Build history of the part. All positions in model axes, mm. A direction names the side the tool comes from. Give positions to 0.01 mm unless a question says otherwise; leave off trailing zeros. Order: outer loops, then holes, each group sorted by start corner. A loop starts at its lowest first (then second) coordinate and runs counter-clockwise, first axis right, second up. Notation, with made-up numbers: (50.5, 27) -> (68.5, 27) arc R30 cw to (68.5, 51) -> close; hole circle Ø4 at (35.25, 87.25). An arc over 180 degrees is marked (long way). Use a Markdown table: item, result. Add a question column.
```python
from build123d import *

# Parameters (mm, degrees)
PAD_DEPTH    = 2.5
PAD001_DEPTH = 1.5
SKETCH002_R  = 2.5
PAD002_DEPTH = 25


with BuildPart() as part:
    # Sketch → Pad (new body, symmetric)
    with BuildSketch(Plane.XY):
        Polygon((-5, 0), (5, 0), (5, -1.284989), (2.784989, -3.5), (-2.784989, -3.5), (-5, -1.284989), align=None)
    extrude(amount=PAD_DEPTH, both=True)

    # Sketch001 → Pad001 (join)
    with BuildSketch(Plane.XZ):
        with BuildLine():
            ThreePointArc((-2.5, 0), (-1.767767, -1.767767), (0, -2.5))
            Line((0, -2.5), (2.5, -2.5))
            Line((2.5, 0), (2.5, -2.5))
            ThreePointArc((2.5, 0), (1.767767, 1.767767), (0, 2.5))
            Line((-2.5, 2.5), (0, 2.5))
            Line((-2.5, 0), (-2.5, 2.5))
        make_face()
    extrude(amount=-PAD001_DEPTH)

    # Sketch002 → Pad002 (join)
    with BuildSketch(Plane.XZ):
        Circle(SKETCH002_R)
    extrude(amount=-PAD002_DEPTH)


solid = part.part
```
(1) Band-saw the part on B-B on x = -1.5. Give the cut face in (y, z).
(2) Band-saw the part on A-A on y = 0.75. Give the cut face in (x, z), plus the area to 3 significant figures.
(3) Band-saw the part on D-D on x = 3.5. Give the cut face in (y, z), plus the area to 3 significant figures.
(4) Wall check: probe 1 along Y at (x, z) = (-1.75, -2); probe 2 along X at (y, z) = (2, 0.4); probe 3 along Y at (x, z) = (3, -1.1). Give the ranges that are in metal, low to high.
(5) Tool access for faces 1 (the face through (2.5, 1, -1)), 2 (the face through (-2, 1.5, 2)), 3 (the face through (-2.5, 1, 1)), 4 (the face through (2, 1.5, -2)), 5 (the face through (4, 0, 0)): list every direction of +Z, -Z, +X, -X, +Y, -Y with a clear straight run to the whole face (end or side of a thin tool).
(6) Band-saw the part on C-C on z = -1.15. Give the cut face in (x, y).
(7) Pin check, flat tips, straight feed: pin 1 Ø1.5 at (x, y) = (-1, 10.5) entering from +Z; pin 2 Ø0.8 at (y, z) = (1, -1.5) entering from +X; pin 3 Ø1 at (y, z) = (7, 1) entering from -X. Stop position of each tip, or through.
Response:
| question | item | result |
|---|---|---|
| 1 | outline | (-3.5, -2.5) -> (0, -2.5) -> (0, -2) -> (25, -2) -> (25, 2) -> (1.5, 2) -> (1.5, 2.5) -> (-3.5, 2.5) -> close |
| 2 | outline | (-2.5, 0) arc R2.5 ccw to (0, -2.5) -> (2.5, -2.5) -> (2.5, 0) arc R2.5 ccw to (0, 2.5) -> (-2.5, 2.5) -> close |
| 2 | area | 22.3 mm² |
| 3 | outline | (-2.78, -2.5) -> (0, -2.5) -> (0, 2.5) -> (-2.78, 2.5) -> close |
| 3 | area | 13.9 mm² |
| 4 | probe 1 | y = -3.5 to 0 |
| 4 | probe 2 | x = -2.47 to 2.47 |
| 4 | probe 3 | y = -3.28 to 0 |
| 5 | face 1 | +Z, -Z, +X, +Y |
| 5 | face 2 | +Z, -X, +Y |
| 5 | face 3 | +Z, -Z, -X, +Y |
| 5 | face 4 | -Z, +X, +Y |
| 5 | face 5 | +Z, +X, +Y |
| 6 | outline | (-5, -1.28) -> (-2.78, -3.5) -> (2.78, -3.5) -> (5, -1.28) -> (5, 0) -> (2.5, 0) -> (2.5, 1.5) -> (2.22, 1.5) -> (2.22, 25) -> (-2.22, 25) -> (-2.22, 0) -> (-5, 0) -> close |
| 7 | pin 1 | stops at z = 2.49 |
| 7 | pin 2 | stops at x = 2.5 |
| 7 | pin 3 | stops at x = -2.45 |
